For this review, take the finished solid that the model builds, in its own axes (mm). Round coordinates to 2 decimals unless told otherwise and drop trailing zeros. Order: outer loops, then holes, each group sorted by start corner. A loop starts at its lowest first (then second) coordinate and runs counter-clockwise, first axis right, second up.
Autodesk Inventor part; units mm, degrees
ref_plane "YZ Plane" through (0, 0, 0) normal (1, 0, 0) x (0, 1, 0)
ref_plane "XZ Plane" through (0, 0, 0) normal (0, 1, 0) x (-1, 0, 0)
ref_plane "XY Plane" through (0, 0, 0) normal (0, 0, 1) x (1, 0, 0)
sketch "スケッチ1" plane through (0, 0, 0) normal (0, 0, 1) x (1, 0, 0)
  circle A0 centre (0, 0) radius 40.5
  dimension "d0" = 81
extrude "プレート1" add sketch "スケッチ1" along normal mid plane 1
sketch "スケッチ2" plane through (0, 0, 0.5) normal (0, 0, 1) x (1, 0, 0)
  circle A0 centre (0, 0) radius 12
  dimension "d2" = 24
extrude "押し出し1" cut sketch "スケッチ2" against normal blind 10
sketch "スケッチ3" plane through (0, 0, 0.5) normal (0, 0, 1) x (1, 0, 0)
  circle A0 centre (0, 0) radius 32
  point P0 (0, 32)
  point P1 (-27.7128, 16)
  point P2 (-27.7128, -16)
  point P3 (0, -32)
  point P4 (27.7128, -16)
  point P5 (27.7128, 16)
  dimension "d5" = 64
  dimension "d8" = 360
hole "穴1" at (0, 32, 0.5) at (-27.7128, 16, 0.5) at (-27.7128, -16, 0.5) at (0, -32, 0.5) at (27.7128, -16, 0.5) at (27.7128, 16, 0.5) direction (0, 0, -1) diameter 4.5 end through all
equation "\"d15\" = Thickness"
equation "\"d1\" = Thickness"
equation "\"BendRadius\" = Thickness"
equation "\"BendReliefWidth\" = Thickness"
equation "\"BendReliefDepth\" = 0.5 * Thickness"
equation "\"CornerReliefSize\" = 4 * Thickness"
equation "\"MinimumRemnant\" = 2 * Thickness"
equation "\"TransitionRadius\" = BendRadius"
equation "\"JacobiRadiusSize\" = BendRadius"
equation "\"GapSize\" = Thickness"
properties part number "unit-plate1" material "CFRP"
(1) Draft analysis for pull direction Y (two halves, no side actions). For faces 1 (the face through (0.86, -34.08, -0.01)), 2 (the face through (8, 10, 0.5)), 3 (the face through (21.77, 34.15, 0.01)), state which applies: pulls with the +Y half, pulls with the -Y half, needs draft (parallel to the pull), parting line crosses it, or undercut.
(2) Add section A-A on y = 0. Give the boundary of the cut face in (x, z), plus the area to 3 significant figures.
(3) Add section C-C on y = 16. Give the boundary of the cut face in (x, z), plus the area to 3 significant figures.
(4) Wall thickness on L1, parallel to X at y = -16, z = -0.1; L2, parallel to X at y = -16.5, z = -0.15; L3, parallel to Y at x = -27, z = -0.2: over which ranges is each line inside the solid? List them lowest first.
(5) Add section B-B on z = -0.25. Give the boundary of the cut face in (x, y).
(6) Clearance check with a flat-ended pin moving along its axis: P1, Ø3.5, axis at x = -27.71, y = 16, coming from the +Z side. State where the tip first meets the part, or that it passes through.
(7) Add section D-D on y = 31. Give the boundary of the cut face in (x, z), plus the area to 3 significant figures.
Here are the results:
1. face 1: undercut
1. face 2: needs draft
1. face 3: parting line crosses it
2. outline: (-40.5, -0.5) - (-12, -0.5) - (-12, 0.5) - (-40.5, 0.5) - close; (12, -0.5) - (40.5, -0.5) - (40.5, 0.5) - (12, 0.5) - close
2. area: 57.0 mm2
3. outline: (-37.21, -0.5) - (-29.96, -0.5) - (-29.96, 0.5) - (-37.21, 0.5) - close; (-25.46, -0.5) - (25.46, -0.5) - (25.46, 0.5) - (-25.46, 0.5) - close; (29.96, -0.5) - (37.21, -0.5) - (37.21, 0.5) - (29.96, 0.5) - close
3. area: 65.4 mm2
4. L1: x = -37.21 to -29.96, -25.46 to 25.46, 29.96 to 37.21
4. L2: x = -36.99 to -29.91, -25.52 to 25.52, 29.91 to 36.99
4. L3: y = -30.19 to -18.13, -13.87 to 13.87, 18.13 to 30.19
5. outline: circle Ø81 at (0, 0); hole circle Ø4.5 at (-27.71, -16); hole circle Ø4.5 at (-27.71, 16); hole circle Ø24 at (0, 0); hole circle Ø4.5 at (0, -32); hole circle Ø4.5 at (0, 32); hole circle Ø4.5 at (27.71, -16); hole circle Ø4.5 at (27.71, 16)
6. P1: passes through
7. outline: (-26.06, -0.5) - (-2.02, -0.5) - (-2.02, 0.5) - (-26.06, 0.5) - close; (2.02, -0.5) - (26.06, -0.5) - (26.06, 0.5) - (2.02, 0.5) - close
7. area: 48.1 mm2
